Input: dimensioned drawing with shaded views. Units: mm. Origin: part minimum x, y, z. A direction names the side the tool comes from. Give positions to 0.01 mm unless a question says otherwise; leave off trailing zeros. Order: outer loops, then holes, each group sorted by start corner. A loop starts at its lowest first (then second) coordinate and runs counter-clockwise, first axis right, second up.
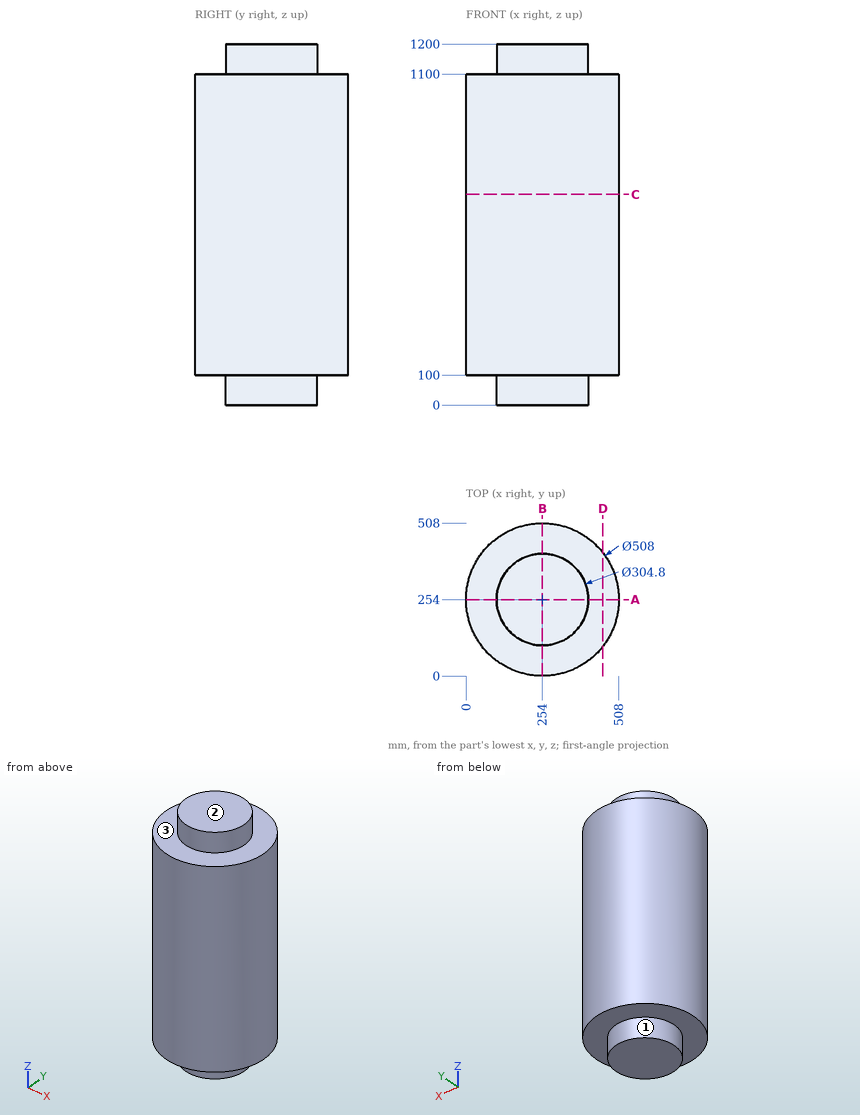
1) Reachability of the marked faces 1, 2 and 3 from +Z, -Z, +X, -X, +Y, -Y: full face, straight path, thin tool, end or side. Return the list, or none.
2) Cut plane D-D (x = 455). Return the cut outline in (y, z), then the cut area to 3 significant figures.
3) Line query: probe 1 along Y at (x, z) = (251, 422.5); probe 2 along Z at (x, y) = (131, 106.5); probe 3 along X at (y, z) = (244, 550.5). Output: solid intervals per line, ascending.
4) First-contact query: P1, Ø2, axis at y = 456.5, z = 347, coming from the +X side; P2, Ø2, axis at x = 342, z = 188.5, coming from the +Y side; P3, Ø2, axis at y = 289, z = 178.5, coming from the -X side. Flat tips, straight axial feed; report the tip coordinate or a pass-through.
5) Cut plane C-C (z = 700.5). Return the cut outline in (x, y), then the cut area to 3 significant figures.
6) Cut plane A-A (y = 254). Return the cut outline in (x, z).
Geometry says:
1. face 1: -Z
1. face 2: +Z, +X, -X, +Y, -Y
1. face 3: +Z
2. outline: (98.71, 100) - (409.29, 100) - (409.29, 1100) - (98.71, 1100) - close
2. area: 311,000 mm2
3. probe 1: y = 0.02 to 507.98
3. probe 2: z = 100 to 1100
3. probe 3: x = 0.2 to 507.8
4. P1: stops at x = 408.64
4. P2: stops at y = 492.64
4. P3: stops at x = 2.29
5. outline: circle Ø508 at (254, 254)
5. area: 203,000 mm2
6. outline: (0, 100) - (101.6, 100) - (101.6, 0) - (406.4, 0) - (406.4, 100) - (508, 100) - (508, 1100) - (406.4, 1100) - (406.4, 1200) - (101.6, 1200) - (101.6, 1100) - (0, 1100) - close
